Check sheet for the drawn part. Datum: minimum x, y, z corner. Units: mm. A direction names the side the tool comes from. Round coordinates to 2 decimals unless told otherwise and drop trailing zeros. Write each loop counter-clockwise with the first axis right and the second up, starting at its lowest first coordinate (ties: lowest second). Pieces come first, ordered by that corner, then holes. Notation, with made-up numbers: (18, 77.25) - (57, 77.25) arc R31 cw to (57, 115.25) - close; hole circle Ø11 at (70, 10.25). An arc over 180 degrees is marked (long way). Answer as a JSON object with one key per item and string values.
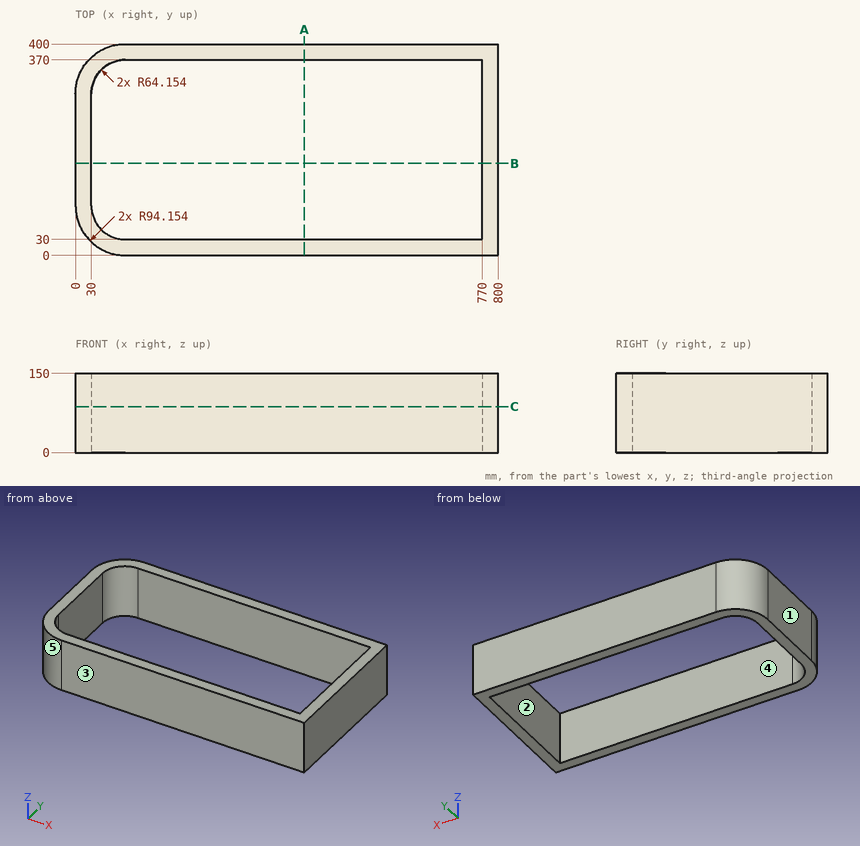
1. Cross-section at A-A (x = 433). Record the boundary of the cut face in (y, z), plus the area to 3 significant figures.
Completed:
{"outline": "(0, 0) - (30, 0) - (30, 150) - (0, 150) - close; (370, 0) - (400, 0) - (400, 150) - (370, 150) - close", "area": "9,000 mm^2"}
2. Material ranges on probe 1 along Y at (x, z) = (479.5, 46); probe 2 along X at (y, z) = (300, 26), recorded low to high. Write a range as from..to.
Completed:
{"probe 1": "y = 0..30, 370..400", "probe 2": "x = 0..30, 770..800"}
3. Cross-section at B-B (y = 174). Record the boundary of the cut face in (x, z).
Completed:
{"outline": "(0, 0) - (30, 0) - (30, 150) - (0, 150) - close; (770, 0) - (800, 0) - (800, 150) - (770, 150) - close"}
4. Mould release check, pull along Y, two halves, no side actions. Record for the marked faces 1, 2 and 3: released by +Y, released by -Y, zero draft, split by the parting line, or undercut.
Completed:
{"face 1": "zero draft", "face 2": "undercut", "face 3": "released by -Y"}
5. Go/stop test with a flat-tipped pin: pin 1 (6 mm diameter, centred on y = 322.5, z = 58, fed in from -X) (1 decimal). Record where the tip stops, or that it passes through.
Completed:
{"pin 1": "stops at x = 1"}
6. Access from +Z, -Z, +X, -X, +Y, -Y to the whole of each face (thin tool, end or side, straight path). Record for the marked faces 4 and 5.
Completed:
{"face 4": "+Z, -Z", "face 5": "+Z, -Z, -X, -Y"}
7. Cross-section at C-C (z = 87). Record the boundary of the cut face in (x, y), plus the area to 3 significant figures.
Completed:
{"outline": "(0, 94.15) arc R94.15 ccw to (94.15, 0) - (800, 0) - (800, 400) - (94.15, 400) arc R94.15 ccw to (0, 305.85) - close; hole (30, 94.15) arc R64.15 ccw to (94.15, 30) - (770, 30) - (770, 370) - (94.15, 370) arc R64.15 ccw to (30, 305.85) - close", "area": "66,400 mm^2"}
